```python
from build123d import *

# Parameters (mm, degrees)
SKETCH1_R                      = 1.6
BOSS_EXTRUDE1_DEPTH            = 3
FILLET1_R                      = 5
FILLET2_R                      = 2
FILLET3_R                      = 1
SKETCH2_R                      = 1.5
SKETCH2_W                      = 8
SKETCH2_H                      = 3
CUT_EXTRUDE1_DEPTH             = 3
FILLET4_R                      = 1
F_2_5_2_5_DIAMETER_HOLE1_D     = 2.5
F_2_5_2_5_DIAMETER_HOLE1_DEPTH = 6
F_2_5_2_5_DIAMETER_HOLE1_TIP   = 0.751075774
SKETCH8_R                      = 1.5
CUT_EXTRUDE2_DEPTH             = 10
SKETCH9_W                      = 3
SKETCH9_H                      = 8
CUT_EXTRUDE3_DEPTH             = 10
FILLET7_R                      = 1


with BuildPart() as part:
    # Sketch1 → Boss-Extrude1 (new body)
    with BuildSketch(Plane.XY):
        with BuildLine():
            Line((20, 75), (-20, 75))
            Line((-20, 75), (-20, -75))
            Line((-20, -75), (-6, -75))
            Line((-6, -75), (-6, -64.219544457))
            ThreePointArc((-6, -64.219544457), (-5.244044241, -45.330460197), (11, -55))
            ThreePointArc((11, -55), (9.669539803, -60.244044241), (6, -64.219544457))
            Line((6, -64.219544457), (6, -75))
            Line((6, -75), (20, -75))
            Line((20, -75), (20, 75))
        make_face()
        with Locations((-15.450283169, -70.450283169)):
            Circle(SKETCH1_R, mode=Mode.SUBTRACT)
        with Locations((-15.450283169, -39.549716831)):
            Circle(SKETCH1_R, mode=Mode.SUBTRACT)
        with Locations((15.450283169, -70.450283169)):
            Circle(SKETCH1_R, mode=Mode.SUBTRACT)
        with Locations((15.450283169, -39.549716831)):
            Circle(SKETCH1_R, mode=Mode.SUBTRACT)
    extrude(amount=BOSS_EXTRUDE1_DEPTH)

    # Fillet1
    fillet1_edges = [part.edges().sort_by_distance(p)[0] for p in [
        (-20, -75, 1.5),
        (-20, 75, 1.5),
        (20, 75, 1.5),
        (20, -75, 1.5),
    ]]
    fillet(fillet1_edges, radius=FILLET1_R)

    # Fillet2
    fillet2_edges = [part.edges().sort_by_distance(p)[0] for p in [
        (-6, -75, 1.5),
        (6, -75, 1.5),
    ]]
    fillet(fillet2_edges, radius=FILLET2_R)

    # Fillet3
    fillet3_edges = [part.edges().sort_by_distance(p)[0] for p in [
        (-6, -64.219544457, 1.5),
        (6, -64.219544457, 1.5),
    ]]
    fillet(fillet3_edges, radius=FILLET3_R)

    # Sketch2 → Cut-Extrude1 (cut)
    with BuildSketch(Plane.XY.offset(3)):
        with Locations((0, -33.5)):
            Circle(SKETCH2_R)
        with Locations((0, 30.5)):
            Circle(SKETCH2_R)
        with Locations((0, 63.5)):
            Circle(SKETCH2_R)
        with Locations((0, -1.5)):
            Circle(SKETCH2_R)
        with Locations((-10, 63.5)):
            Rectangle(SKETCH2_W, SKETCH2_H)
        with Locations((10, 63.5)):
            Rectangle(SKETCH2_W, SKETCH2_H)
        with Locations((-10, 30.5)):
            Rectangle(SKETCH2_W, SKETCH2_H)
        with Locations((10, 30.5)):
            Rectangle(SKETCH2_W, SKETCH2_H)
        with Locations((-10, -33.5)):
            Rectangle(SKETCH2_W, SKETCH2_H)
        with Locations((10, -33.5)):
            Rectangle(SKETCH2_W, SKETCH2_H)
    extrude(amount=-CUT_EXTRUDE1_DEPTH, mode=Mode.SUBTRACT)

    # Fillet4
    fillet4_edges = [part.edges().sort_by_distance(p)[0] for p in [
        (14, -32, 1.5),
        (14, -35, 1.5),
        (6, -35, 1.5),
        (6, -32, 1.5),
        (14, 32, 1.5),
        (14, 29, 1.5),
        (6, 29, 1.5),
        (6, 32, 1.5),
        (-6, 32, 1.5),
        (-6, 29, 1.5),
        (-14, 29, 1.5),
        (-14, 32, 1.5),
        (-6, 65, 1.5),
        (-6, 62, 1.5),
        (-14, 62, 1.5),
        (-14, 65, 1.5),
        (14, 65, 1.5),
        (14, 62, 1.5),
        (6, 62, 1.5),
        (6, 65, 1.5),
        (-6, -32, 1.5),
        (-6, -35, 1.5),
        (-14, -35, 1.5),
        (-14, -32, 1.5),
    ]]
    fillet(fillet4_edges, radius=FILLET4_R)

    # Ø2.5 (2.5) Diameter Hole1
    with Locations(Plane.XY.offset(3)):
        with Locations((14, -17.5), (-14, -17.5), (-14, 14.5), (14, 14.5), (14, 47), (-14, 47)):
            Hole(F_2_5_2_5_DIAMETER_HOLE1_D / 2, depth=F_2_5_2_5_DIAMETER_HOLE1_DEPTH)
            with Locations((0, 0, -(F_2_5_2_5_DIAMETER_HOLE1_DEPTH + F_2_5_2_5_DIAMETER_HOLE1_TIP / 2))):  # 118° drill point
                Cone(0, F_2_5_2_5_DIAMETER_HOLE1_D / 2, F_2_5_2_5_DIAMETER_HOLE1_TIP, mode=Mode.SUBTRACT)

    # Sketch8 → Cut-Extrude2 (cut)
    with BuildSketch(Plane.XY.offset(3)):
        with Locations((-14, 70)):
            Circle(SKETCH8_R)
        with Locations((14, 70)):
            Circle(SKETCH8_R)
    extrude(amount=-CUT_EXTRUDE2_DEPTH, mode=Mode.SUBTRACT)

    # Sketch9 → Cut-Extrude3 (cut)
    with BuildSketch(Plane.XY.offset(3)):
        with Locations((0, -16.75)):
            Rectangle(SKETCH9_W, SKETCH9_H)
        with Locations((0, 13.75)):
            Rectangle(SKETCH9_W, SKETCH9_H)
    extrude(amount=-CUT_EXTRUDE3_DEPTH, mode=Mode.SUBTRACT)

    # Fillet7
    fillet7_edges = [part.edges().sort_by_distance(p)[0] for p in [
        (1.5, 17.75, 1.5),
        (1.5, 9.75, 1.5),
        (-1.5, 9.75, 1.5),
        (-1.5, 17.75, 1.5),
        (-1.5, -20.75, 1.5),
        (-1.5, -12.75, 1.5),
        (1.5, -12.75, 1.5),
        (1.5, -20.75, 1.5),
    ]]
    fillet(fillet7_edges, radius=FILLET7_R)


solid = part.part
```
Work out the finished part from the listing and answer in its coordinate system (mm). A direction names the side the tool comes from. Coordinates: 2 decimals unless noted, no trailing zeros. Write each loop counter-clockwise with the first axis right and the second up, starting at its lowest first coordinate (ties: lowest second). Pieces come first, ordered by that corner, then holes. Notation, with made-up numbers: (13.25, -25.5) - (50.25, -25.5) arc R13 ccw to (50.25, -21.5) - close; hole circle Ø3 at (-37, -9). An arc over 180 degrees is marked (long way). Answer as a JSON object with one key per item and string values.
Q1. Find section D-D (z = 2.15). State how many separate pieces and enclosed holes the cut face has, plus the area to 3 significant figures.
Results list:
{"separate pieces": "1", "enclosed holes": "24", "area": "5,190 mm^2"}
Q2. For a pull along Y with two mould halves and no side action, classify faces 1 (the cylindrical face through (13.805, 71.487, 1.521)), 2 (the flat face through (-5, 18, 3)), 3 (the flat face through (10, 62, 2)), 4 (the flat face through (0, 75, 1)) as pulls with the +Y half, pulls with the -Y half, needs draft (parallel to the pull), parting line crosses it, or undercut.
Results list:
{"face 1": "undercut", "face 2": "needs draft", "face 3": "undercut", "face 4": "pulls with the +Y half"}
Q3. Find section C-C (y = 14.5). Write down the section's boundary in (x, z), plus the area to 3 significant figures.
Results list:
{"outline": "(-20, 0) - (-15.25, 0) - (-15.25, 3) - (-20, 3) - close; (-12.75, 0) - (-1.5, 0) - (-1.5, 3) - (-12.75, 3) - close; (1.5, 0) - (12.75, 0) - (12.75, 3) - (1.5, 3) - close; (15.25, 0) - (20, 0) - (20, 3) - (15.25, 3) - close", "area": "96.0 mm^2"}
Q4. Find section B-B (y = -1.5). Write down the section's boundary in (x, z), plus the area to 3 significant figures.
Results list:
{"outline": "(-20, 0) - (-1.5, 0) - (-1.5, 3) - (-20, 3) - close; (1.5, 0) - (20, 0) - (20, 3) - (1.5, 3) - close", "area": "111 mm^2"}
Q5. Consider L1, parallel to Y at x = 11.5, z = 1.85; L2, parallel to X at y = 70, z = 2.15; L3, parallel to Y at x = 16.5, z = 0.6. Determine where each line is inside the solid, lowest interval first. Write a range as from..to.
Results list:
{"L1": "y = -75..-35, -32..29, 32..62, 65..75", "L2": "x = -20..-15.5, -12.5..12.5, 15.5..20", "L3": "y = -74.77..-71.66, -69.24..-40.76, -38.34..74.77"}
Q6. Which of the six approach directions +Z, -Z, +X, -X, +Y, -Y give full straight-line access (tool end or side, diameter ignored) to faces 5 (the flat face through (-20, 1, 1)), 6 (the flat face through (1.5, 14, 2)), 7 (the flat face through (6, -69, 1))?
Results list:
{"face 5": "+Z, -Z, -X, +Y, -Y", "face 6": "+Z, -Z", "face 7": "+Z, -Z, -Y"}
Q7. Find section A-A (y = 47). Write down the section's boundary in (x, z).
Results list:
{"outline": "(-20, 0) - (-15.25, 0) - (-15.25, 3) - (-20, 3) - close; (-12.75, 0) - (12.75, 0) - (12.75, 3) - (-12.75, 3) - close; (15.25, 0) - (20, 0) - (20, 3) - (15.25, 3) - close"}
Q8. Given pin 1 Ø3 at (x, y) = (14, 47) entering from +Z; pin 2 Ø1.5 at (x, z) = (2.5, 2) entering from -Y, each flat-ended and moving along its own axis, determine where each tip first touches the part or whether it passes through.
Results list:
{"pin 1": "stops at z = 3", "pin 2": "stops at y = -44.49"}
